CAD build for the part. Positions are in the model's coordinates, mm. Face numbers are marked on the shaded views. Round coordinates to 2 decimals unless told otherwise and drop trailing zeros. Order: outer loops, then holes, each group sorted by start corner. A loop starts at its lowest first (then second) coordinate and runs counter-clockwise, first axis right, second up. Notation, with made-up numbers: M 84,39 L 117,39 A16 cw 117,64 Z; hole C -9.75,61.25 d4. An arc over 180 degrees is marked long. Answer as a JSON object with one key per item and string values. Group by question number.
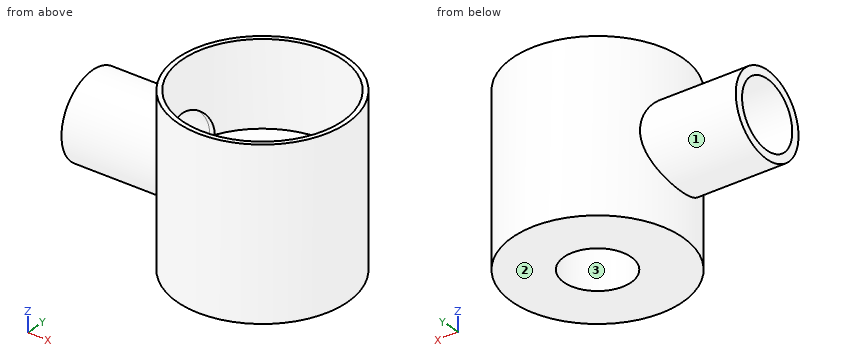
```python
from build123d import *

# Parameters (mm, degrees)
F0_R     = 50.8
F0_R_2   = 48
F1_DEPTH = 50
F2_R     = 50.8
F2_R_2   = 20.0025
F3_DEPTH = 50
F4_R     = 20
F5_DEPTH = 50.801
F7_R     = 25
F7_R_2   = 20


with BuildPart() as f1:
    # F0 (on Top) → F1 (new body, symmetric)
    with BuildSketch(Plane.XY):
        Circle(F0_R)
        Circle(F0_R_2, mode=Mode.SUBTRACT)
    extrude(amount=F1_DEPTH, both=True)

    # F2 (on Top) → F3 (join, through all)
    with BuildSketch(Plane.XY):
        Circle(F2_R)
        Circle(F2_R_2, mode=Mode.SUBTRACT)
    extrude(amount=-F3_DEPTH)

    # F4 (on Right) → F5 (cut, through all)
    with BuildSketch(Plane.YZ):
        Circle(F4_R)
    extrude(amount=-F5_DEPTH, mode=Mode.SUBTRACT)

    # F7 (on offset) → F8 (join, up to the next surface of F1)
    with BuildSketch(Plane.YZ.offset(-101.6)):
        Circle(F7_R)
        Circle(F7_R_2, mode=Mode.SUBTRACT)
    extrude(until=Until.NEXT)


solid = f1.part
```
Item 1: Cut at A-A, the plane y = 0. Give the cut face in (x, z), and give its area (3 significant figures).
Item 2: Flat gauge pins, fed straight in: pin 1 Ø1 at (y, z) = (12, -23.5) entering from +X; pin 2 Ø5 at (x, y) = (-30, -25.5) entering from +Z; pin 3 Ø3 at (y, z) = (39, -10) entering from -X; pin 4 Ø12 at (y, z) = (12.5, 8) entering from -X. Where does each tip first touch, or does it go through?
Item 3: Drill centre lines: line 1 (Y direction, x = 0, z = 32); line 2 (Y direction, x = -64, z = 0). Where is each one in solid material? Low to high. Write a range as [from, to].
Item 4: Cut at C-C, the plane x = -22.5. Give the cut face in (y, z).
Item 5: Cut at D-D, the plane z = 15.5. Give the cut face in (x, y), and give its area (3 significant figures).
Item 6: Two-plate mould, pull along Y, no slides. Class the marked faces 1, 2 and 3: +Y half, -Y half, draft (parallel to the pull), parting line (faces both ways), or undercut.
Item 7: Cut at B-B, the plane x = 5. Give the cut face in (y, z), and give its area (3 significant figures).
Response values:
{
 "1": {"outline": "M -101.6,-25 L -50.8,-25 L -50.8,-50 L -20,-50 L -20,-20 L -101.6,-20 Z; M -101.6,20 L -48,20 L -48,50 L -50.8,50 L -50.8,25 L -101.6,25 Z; M 20,-50 L 50.8,-50 L 50.8,50 L 48,50 L 48,0 L 20,0 Z", "area": "3,200 mm^2"},
 "2": {"pin 1": "x = 49.48", "pin 2": "z = 0", "pin 3": "x = -34.27", "pin 4": "x = -101.6"},
 "3": {"line 1": "[-50.8, -48], [48, 50.8]", "line 2": "[-25, -20], [20, 25]"},
 "4": {"outline": "M -45.55,-50 L 45.55,-50 L 45.55,50 L 42.4,50 L 42.4,0 L 20,0 A20 cw -20,0 L -42.4,0 L -42.4,50 L -45.55,50 Z"},
 "5": {"outline": "M -101.6,-19.62 L -46.86,-19.62 A50.8 ccw long -46.86,19.62 L -101.6,19.62 L -101.6,12.64 L -46.31,12.64 A48 cw long -46.31,-12.64 L -101.6,-12.64 Z", "area": "1,540 mm^2"},
 "6": {"face 1": "parting line", "face 2": "draft", "face 3": "undercut"},
 "7": {"outline": "M -50.55,-50 L -19.37,-50 L -19.37,0 L -47.74,0 L -47.74,50 L -50.55,50 Z; M 19.37,-50 L 50.55,-50 L 50.55,50 L 47.74,50 L 47.74,0 L 19.37,0 Z", "area": "3,400 mm^2"}
}
